The listing builds one solid part. Answer for the finished solid, in the listing's coordinates (mm). A direction names the side the tool comes from. Give positions to 0.01 mm unless a question says otherwise; leave off trailing zeros. Write each loop counter-clockwise with the first axis right and the second up, starting at its lowest first coordinate (ties: lowest second). Pieces come first, ordered by that corner, then holes. Notation, with made-up numbers: M 30.25,51 L 58.25,51 A20 ccw 58.25,76 Z; hole C 70,74 d11. An arc over 180 degrees is marked long. Answer as a JSON object with one key per item and string values.
```python
from build123d import *

# Parameters (mm, degrees)
SKETCH1_R                                      = 16.891
BOSS_EXTRUDE1_DEPTH                            = 56.0324
SKETCH9_R                                      = 9.525
CUT_EXTRUDE6_DEPTH                             = 61.911752657
SKETCH10_R                                     = 11.43
BOSS_EXTRUDE2_DEPTH                            = 19.05
CUT_EXTRUDE7_START                             = -52.06365
SKETCH11_R                                     = 9.525
CUT_EXTRUDE7_DEPTH                             = 52.06365
CUT_EXTRUDE8_START                             = -3.96875
CUT_EXTRUDE8_DEPTH                             = 3.96875
CSK_FOR_2_FLAT_HEAD_MACHINE_SCREW1_D           = 2.2606
CSK_FOR_2_FLAT_HEAD_MACHINE_SCREW1_CSINK_D     = 4.3688
CSK_FOR_2_FLAT_HEAD_MACHINE_SCREW1_CSINK_ANGLE = 82
CIRPATTERN1_COUNT                              = 6
F_1_2_0_4_DIAMETER_HOLE1_D                     = 10.16
F_1_2_0_4_DIAMETER_HOLE1_DEPTH                 = 12.7
F_1_2_0_4_DIAMETER_HOLE1_TIP                   = 3.052371945
FILLET1_R                                      = 1.27
CUT_EXTRUDE9_START                             = -12.7
SKETCH17_W                                     = 16.51
SKETCH17_H                                     = 16.51
CUT_EXTRUDE9_DEPTH                             = 12.7


with BuildPart() as part:
    # Sketch1 → Boss-Extrude1 (new body)
    with BuildSketch(Plane.XY):
        Circle(SKETCH1_R)
    extrude(amount=BOSS_EXTRUDE1_DEPTH)

    # Sketch9 → Cut-Extrude6 (cut, through all)
    with BuildSketch(Plane(origin=(0, 0, 0), x_dir=(-1, 0, 0), z_dir=(0, 0, -1))):
        Circle(SKETCH9_R)
        with BuildLine():
            ThreePointArc((-5.359640753, -7.874), (0, -9.525), (5.359640753, -7.874))
            Line((5.359640753, -7.874), (-5.359640753, -7.874))
        make_face()
        with BuildLine():
            ThreePointArc((-7.874, 5.359640753), (-9.525, 0), (-7.874, -5.359640753))
            Line((-7.874, -5.359640753), (-7.874, 5.359640753))
        make_face()
        with BuildLine():
            Line((-5.359640753, 7.874), (5.359640753, 7.874))
            ThreePointArc((5.359640753, 7.874), (0, 9.525), (-5.359640753, 7.874))
        make_face()
        with BuildLine():
            Line((7.874, 5.359640753), (7.874, -5.359640753))
            ThreePointArc((7.874, -5.359640753), (9.102897204, -2.804084075), (9.525, 0))
            ThreePointArc((9.525, 0), (9.102897204, 2.804084075), (7.874, 5.359640753))
        make_face()
    extrude(amount=-CUT_EXTRUDE6_DEPTH, mode=Mode.SUBTRACT)

    # Sketch10 → Boss-Extrude2 (add)
    # profile 1 of 2: a face of its own
    with BuildSketch(Plane(origin=(0, 0, 0), x_dir=(-1, 0, 0), z_dir=(0, 0, -1))):
        Circle(SKETCH10_R)
        with BuildLine():
            ThreePointArc((-5.359640753, -7.874), (-4.453933477, 8.419507206), (9.525, 0))
            ThreePointArc((9.525, 0), (8.419507206, -4.453933477), (5.359640753, -7.874))
            ThreePointArc((5.359640753, -7.874), (0, -9.525), (-5.359640753, -7.874))
        make_face(mode=Mode.SUBTRACT)
    # profile 2 of 2: a face of its own
    with BuildSketch(Plane(origin=(0, 0, 0), x_dir=(-1, 0, 0), z_dir=(0, 0, -1))):
        Circle(SKETCH10_R)
        with BuildLine():
            ThreePointArc((-5.359640753, -7.874), (-4.453933477, 8.419507206), (9.525, 0))
            ThreePointArc((9.525, 0), (8.419507206, -4.453933477), (5.359640753, -7.874))
            ThreePointArc((5.359640753, -7.874), (0, -9.525), (-5.359640753, -7.874))
        make_face(mode=Mode.SUBTRACT)
    extrude(amount=-BOSS_EXTRUDE2_DEPTH)

    # Sketch11 → Cut-Extrude7 (cut)
    with BuildSketch(Plane.XY.offset(56.0324).offset(CUT_EXTRUDE7_START)):
        with BuildLine():
            Line((-9.153468369, -2.634319991), (-10.984162043, -3.161183989))
            ThreePointArc((-10.984162043, -3.161183989), (1.596234295, -11.317991698), (11.43, 0))
            ThreePointArc((11.43, 0), (1.610471515, 11.315974615), (-10.976173491, 3.188810986))
            Line((-10.976173491, 3.188810986), (-9.146811242, 2.657342489))
            ThreePointArc((-9.146811242, 2.657342489), (1.342059596, 9.429978846), (9.525, 0))
            ThreePointArc((9.525, 0), (1.330195246, -9.431659748), (-9.153468369, -2.634319991))
        make_face()
        with Locations(Location((0, 0, 0), (0, 0, 180))):
            Circle(SKETCH11_R)
        with BuildLine():
            ThreePointArc((-10.984162043, -3.161183989), (-11.297244321, 0.014212394), (-10.976173491, 3.188810986))
            Line((-10.976173491, 3.188810986), (0, 0))
            Line((0, 0), (-10.984162043, -3.161183989))
        make_face()
        with BuildLine():
            ThreePointArc((-10.976173491, 3.188810986), (-11.429990955, 0.014379395), (-10.984162043, -3.161183989))
            ThreePointArc((-10.984162043, -3.161183989), (-11.297244321, 0.014212394), (-10.976173491, 3.188810986))
        make_face()
    extrude(amount=CUT_EXTRUDE7_DEPTH, mode=Mode.SUBTRACT)

    # Sketch11<4> → Cut-Extrude8 (cut)
    with BuildSketch(Plane.XY.offset(56.0324).offset(CUT_EXTRUDE8_START)):
        with BuildLine():
            ThreePointArc((-10.976173491, 3.188810986), (-11.297244321, 0.014212394), (-10.984162043, -3.161183989))
            Line((-10.984162043, -3.161183989), (0, 0))
            Line((0, 0), (-10.976173491, 3.188810986))
        make_face()
        with BuildLine():
            ThreePointArc((-10.976173491, 3.188810986), (-11.429990955, 0.014379395), (-10.984162043, -3.161183989))
            ThreePointArc((-10.984162043, -3.161183989), (-11.297244321, 0.014212394), (-10.976173491, 3.188810986))
        make_face()
        with BuildLine():
            Line((-16.232150575, -4.67152745), (-10.984162043, -3.161183989))
            ThreePointArc((-10.984162043, -3.161183989), (-11.429990955, 0.014379395), (-10.976173491, 3.188810986))
            Line((-10.976173491, 3.188810986), (-16.220345269, 4.712354013))
            ThreePointArc((-16.220345269, 4.712354013), (-16.925737574, 0.021293268), (-16.232150575, -4.67152745))
        make_face()
        with BuildLine():
            Line((0, 0), (-10.984162043, -3.161183989))
            ThreePointArc((-10.984162043, -3.161183989), (1.596234295, -11.317991698), (11.43, 0))
            ThreePointArc((11.43, 0), (1.610471515, 11.315974615), (-10.976173491, 3.188810986))
            Line((-10.976173491, 3.188810986), (0, 0))
        make_face()
    cut_extrude8 = extrude(amount=CUT_EXTRUDE8_DEPTH, mode=Mode.SUBTRACT)

    # CSK for #2 Flat Head Machine Screw1 (through all)
    with Locations(Plane(origin=(0, 0, 0), x_dir=(-1, 0, 0), z_dir=(0, 0, -1))):
        with Locations((11.671937945, 6.75838911)):
            csk_for_2_flat_head_machine_screw1 = CounterSinkHole(CSK_FOR_2_FLAT_HEAD_MACHINE_SCREW1_D / 2, CSK_FOR_2_FLAT_HEAD_MACHINE_SCREW1_CSINK_D / 2, counter_sink_angle=CSK_FOR_2_FLAT_HEAD_MACHINE_SCREW1_CSINK_ANGLE)

    # CirPattern1: Cut-Extrude8, CSK for #2 Flat Head Machine Screw1 ×6 about axis
    cirpattern1_axis = Axis((0, 0, 0), (0, 0, 1))
    add([cut_extrude8.rotate(cirpattern1_axis, i * 360 / CIRPATTERN1_COUNT) for i in range(1, CIRPATTERN1_COUNT)], mode=Mode.SUBTRACT)
    add([csk_for_2_flat_head_machine_screw1.rotate(cirpattern1_axis, i * 360 / CIRPATTERN1_COUNT) for i in range(1, CIRPATTERN1_COUNT)], mode=Mode.SUBTRACT)

    # 1/2 (0.4) Diameter Hole1
    with Locations(Plane(origin=(16.890986634, -0.02124955, 39.36365), x_dir=(0.001258039772, 0.999999208668, 0), z_dir=(0.999999208668, -0.001258039772, 0))):
        with Locations((0, 0)):
            Hole(F_1_2_0_4_DIAMETER_HOLE1_D / 2, depth=F_1_2_0_4_DIAMETER_HOLE1_DEPTH)
            with Locations((0, 0, -(F_1_2_0_4_DIAMETER_HOLE1_DEPTH + F_1_2_0_4_DIAMETER_HOLE1_TIP / 2))):  # 118° drill point
                Cone(0, F_1_2_0_4_DIAMETER_HOLE1_D / 2, F_1_2_0_4_DIAMETER_HOLE1_TIP, mode=Mode.SUBTRACT)

    # Fillet1
    # the kernel refuses this fillet: 1.27 mm, written as the material it takes off along each edge
    with BuildSketch(Plane(origin=(0, 0, 0), x_dir=(1, 0, 0), z_dir=(0, -1, 0))) as fillet1_piece_1:
        with BuildLine():
            CenterArc((16.891 - FILLET1_R, FILLET1_R), FILLET1_R, 270, 90)
            Line((16.891 - FILLET1_R, 0), (16.891, 0))
            Line((16.891, 0), (16.891, FILLET1_R))
        make_face()
    revolve(axis=Axis((0, 0, 0), (0, 0, 1)), mode=Mode.SUBTRACT)

    # Sketch17 → Cut-Extrude9 (cut)
    with BuildSketch(Plane(origin=(0, 0, 0), x_dir=(-1, 0, 0), z_dir=(0, 0, -1)).offset(CUT_EXTRUDE9_START)):
        with Locations((-0.016967686, 0.019651839)):
            Rectangle(SKETCH17_W, SKETCH17_H)
    extrude(amount=CUT_EXTRUDE9_DEPTH, mode=Mode.SUBTRACT)


solid = part.part
```
1. Flat-ended cylindrical pins translate along their axes: pin 1 (3 mm diameter, centred on x = -5.5, z = 3, fed in from -Y); pin 2 (2 mm diameter, centred on y = 10, z = 24.5, fed in from +X); pin 3 (2.5 mm diameter, centred on x = -0.02, y = -13.49, fed in from -Z); pin 4 (4.5 mm diameter, centred on x = 13.5, y = 2, fed in from +Z). Find the tip coordinate at first contact, or state that the pin passes through.
Verdict:
{"pin 1": "stops at y = -16.41", "pin 2": "stops at x = 14.29", "pin 3": "stops at z = 1.07", "pin 4": "stops at z = 56.03"}
2. A cutting plane is placed at C-C, the plane y = -1.5. Count the separate pieces of the cut face and the enclosed holes in it, plus the area to 3 significant figures.
Verdict:
{"separate pieces": "3", "enclosed holes": "0", "area": "533 mm2"}
3. The mould has two halves that part along X. Classify faces 1 (the flat face through (-13.645, -3.927, 54.02)), 2 (the flat face through (-13, 7, 56.032)), 3 (the flat face through (0, 10, 3.969)), 4 (the flat face through (13.645, 3.927, 54.02)): released by +X, released by -X, zero draft, split by the parting line, or undercut.
Verdict:
{"face 1": "released by -X", "face 2": "zero draft", "face 3": "undercut", "face 4": "released by +X"}
4. A cutting plane is placed at A-A, the plane z = 41.5. Give the vertices of the cut face in (x, y).
Verdict:
{"outline": "M 10.45,-4.62 A11.43 cw long 10.47,4.6 L 16.26,4.59 A16.89 ccw long 16.24,-4.63 Z; hole C -11.69,-6.73 d2.26; hole C -11.67,6.76 d2.26; hole C -0.02,-13.49 d2.26; hole C 0.02,13.49 d2.26; hole C 11.67,-6.76 d2.26; hole C 11.69,6.73 d2.26"}
5. A cutting plane is placed at B-B, the plane z = 14. Give the vertices of the cut face in (x, y).
Verdict:
{"outline": "C 0,0 d33.78; hole C -11.69,-6.73 d2.26; hole C -11.67,6.76 d2.26; hole C 0,0 d22.86; hole C -0.02,-13.49 d2.26; hole C 0.02,13.49 d2.26; hole C 11.67,-6.76 d2.26; hole C 11.69,6.73 d2.26"}
6. Consider line 1 along X through (y, z) = (6.5, 29.5); line 2 along X through (y, z) = (7.5, 12.5); line 3 along Z through (x, y) = (10, -4.5). Determine where each line is inside the solid, lowest interval first.
Verdict:
{"line 1": "x = -15.59 to -12.77, -10.57 to -9.4, 9.4 to 10.58, 12.8 to 15.59", "line 2": "x = -15.13 to -12.52, -10.82 to -8.63, 8.63 to 10.86, 12.52 to 15.13", "line 3": "z = 0 to 3.97"}
7. For faces 5 (the flat face through (-10.19, -9.77, 54.02)), 6 (the flat face through (10.19, 9.77, 54.02)), 7 (the flat face through (10, 0, 3.969)), 8 (the flat face through (-6.9, -8.235, 3.6)), 9 (the cylindrical face through (12.57, -6.07, 29.01)), determine the directions among +Z, -Z, +X, -X, +Y, -Y from which every point of the face is accessible in a straight line to the end or side of a thin tool.
Verdict:
{"face 5": "+Z, -Y", "face 6": "+Z, +Y", "face 7": "+Z", "face 8": "-Z", "face 9": "+Z, -Z"}
